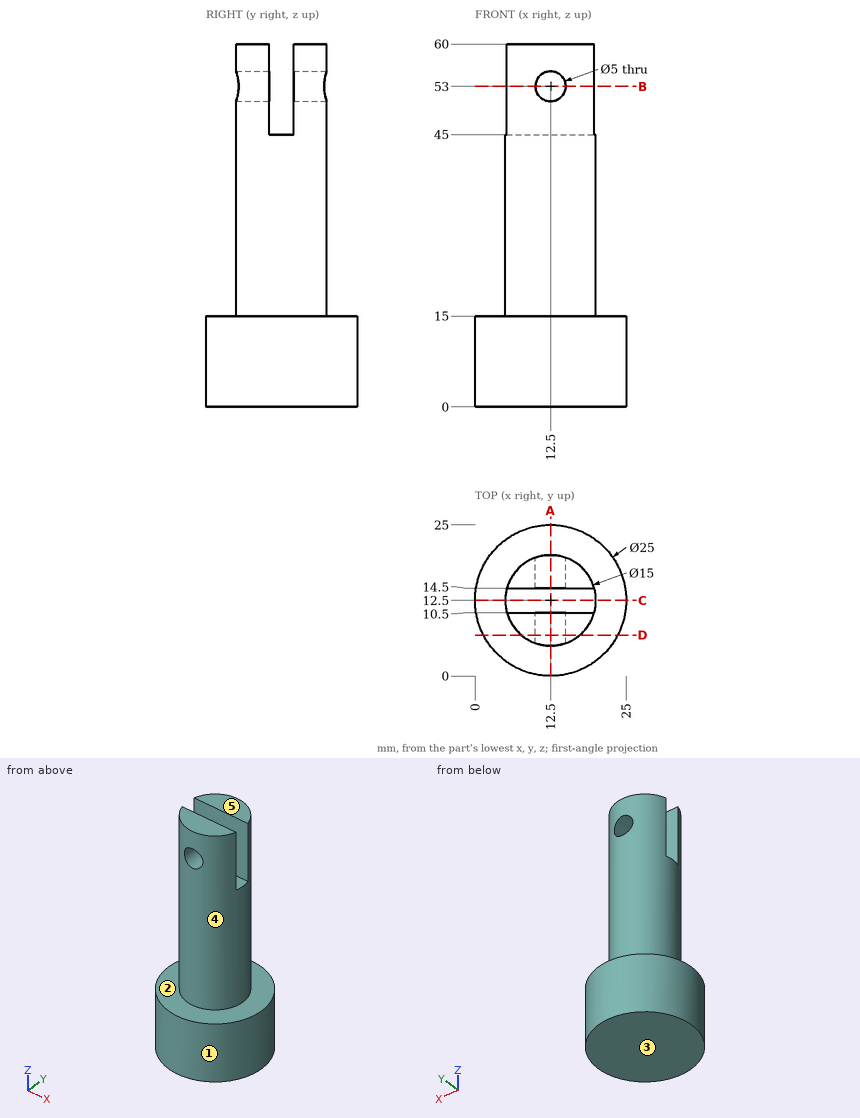
Check sheet for the drawn part. Datum: minimum x, y, z corner. Units: mm. A direction names the side the tool comes from. Round coordinates to 2 decimals unless told otherwise and drop trailing zeros. Write each loop counter-clockwise with the first axis right and the second up, starting at its lowest first coordinate (ties: lowest second). Pieces come first, ordered by that corner, then holes. Notation, with made-up numbers: (-31.75, -20) - (26.25, -20) arc R24 cw to (26.25, 11) - close; hole circle Ø3 at (-13, 17.5). An arc over 180 degrees is marked (long way). Write each question's results on one line, items separated by ' | '.
(1) Depth check by flat-ended pin: pin 1 Ø1.5 at (x, z) = (10.5, 51.5) entering from +Y; pin 2 Ø7 at (x, z) = (10, 49) entering from +Y; pin 3 Ø4 at (x, z) = (12.5, 53) entering from +Y; pin 4 Ø1 at (x, y) = (17, 4) entering from +Z. Enter the tip coordinate at first touch or a pass-through.
Computed:
pin 1: stops at y = 19.86 | pin 2: stops at y = 20 | pin 3: passes through | pin 4: stops at z = 15
(2) Draft check along Z on the marked faces 1, 2 and 3. Enter one of: pulls with the +Z half, pulls with the -Z half, needs draft (parallel to the pull), parting line crosses it, or undercut.
Computed:
face 1: needs draft | face 2: pulls with the +Z half | face 3: pulls with the -Z half
(3) Sectioned sample at B-B, the plane z = 53. Enter the section's corners in (x, y), plus the area to 3 significant figures.
Computed:
outline: (5.27, 10.5) arc R7.5 ccw to (10, 5.43) - (10, 10.5) - close; (5.27, 14.5) - (10, 14.5) - (10, 19.57) arc R7.5 ccw to start; (15, 5.43) arc R7.5 ccw to (19.73, 10.5) - (15, 10.5) - close; (15, 14.5) - (19.73, 14.5) arc R7.5 ccw to (15, 19.57) - close | area: 63.8 mm^2
(4) Set-up check for the marked faces 4 and 5: record each of +Z, -Z, +X, -X, +Y, -Y from which the full face is reachable in a straight line by a thin tool's end or side.
Computed:
face 4: +Z | face 5: +Z, +X, -X, +Y, -Y
(5) Sectioned sample at D-D, the plane y = 6.75. Enter the section's corners in (x, z).
Computed:
outline: (1.4, 0) - (23.6, 0) - (23.6, 15) - (17.32, 15) - (17.32, 60) - (7.68, 60) - (7.68, 15) - (1.4, 15) - close; hole circle Ø5 at (12.5, 53)
(6) Thickness scan on probe 1 along Z at (x, y) = (12.5, 7.9); probe 2 along Z at (x, y) = (22.5, 16.75); probe 3 along Z at (x, y) = (14.5, 14). Record the ranges inside material, lowest first. Write a range as from..to.
Computed:
probe 1: z = 0..50.5, 55.5..60 | probe 2: z = 0..15 | probe 3: z = 0..45
(7) Sectioned sample at A-A, the plane x = 12.5. Enter the section's corners in (y, z).
Computed:
outline: (0, 0) - (25, 0) - (25, 15) - (20, 15) - (20, 50.5) - (14.5, 50.5) - (14.5, 45) - (10.5, 45) - (10.5, 50.5) - (5, 50.5) - (5, 15) - (0, 15) - close; (5, 55.5) - (10.5, 55.5) - (10.5, 60) - (5, 60) - close; (14.5, 55.5) - (20, 55.5) - (20, 60) - (14.5, 60) - close
(8) Sectioned sample at C-C, the plane y = 12.5. Enter the section's corners in (x, z).
Computed:
outline: (0, 0) - (25, 0) - (25, 15) - (20, 15) - (20, 45) - (5, 45) - (5, 15) - (0, 15) - close
